from build123d import *

# Parameters (mm, degrees)
SKETCH2_R               = 3.175
BOSS_EXTRUDE2_DEPTH     = 3.81
SKETCH1_R               = 3.175
BOSS_EXTRUDE3_DEPTH     = 3.81
CUT_EXTRUDE1_DEPTH      = 130.839106153
CUT_EXTRUDE1_DEPTH_BACK = 130.839106153
SKETCH3_R               = 3.175


with BuildPart() as part:
    # Sketch2 → Boss-Extrude2 (new body)
    with BuildSketch(Plane(origin=(0, 0, 0), x_dir=(1, 0, 0), z_dir=(0, 1, 0))):
        with BuildLine():
            Line((-45.85683296, -6.1921984), (-122.640093118, 11.252530303))
            ThreePointArc((-122.640093118, 11.252530303), (-127.425458558, 18.851561662), (-119.826427198, 23.636927102))
            Line((-119.826427198, 23.636927102), (-43.04316704, 6.1921984))
            ThreePointArc((-43.04316704, 6.1921984), (-38.2578016, -1.40683296), (-45.85683296, -6.1921984))
        make_face()
        with Locations(Location((-121.233260158, 17.444728703, 0), (0, 0, 90))):
            Circle(SKETCH2_R, mode=Mode.SUBTRACT)
    extrude(amount=BOSS_EXTRUDE2_DEPTH)

    # Sketch1 → Boss-Extrude3 (add)
    with BuildSketch(Plane(origin=(0, 0, 0), x_dir=(1, 0, 0), z_dir=(0, 1, 0))):
        with BuildLine():
            Line((-44.45, 6.35), (44.45, 6.35))
            ThreePointArc((44.45, 6.35), (50.8, 0), (44.45, -6.35))
            Line((44.45, -6.35), (-44.45, -6.35))
            ThreePointArc((-44.45, -6.35), (-50.8, 0), (-44.45, 6.35))
        make_face()
        with Locations(Location((44.45, 0, 0), (0, 0, 90))):
            Circle(SKETCH1_R, mode=Mode.SUBTRACT)
    extrude(amount=BOSS_EXTRUDE3_DEPTH)

    # Sketch3 → Cut-Extrude1 (cut, two sides: drawn at the far end of the back side and taken through both)
    with BuildSketch(Plane(origin=(0, 3.81, 0), x_dir=(1, 0, 0), z_dir=(0, 1, 0)).offset(-CUT_EXTRUDE1_DEPTH_BACK)):
        with Locations(Location((-44.45, 0, 0), (0, 0, 270))):
            Circle(SKETCH3_R)
    extrude(amount=CUT_EXTRUDE1_DEPTH + CUT_EXTRUDE1_DEPTH_BACK, mode=Mode.SUBTRACT)


solid = part.part
Here's how the part is built. I have some questions about the finished solid (model axes, mm). A direction names the side the tool comes from. Coordinates: 2 decimals unless noted, no trailing zeros. Write each loop counter-clockwise with the first axis right and the second up, starting at its lowest first coordinate (ties: lowest second). Pieces come first, ordered by that corner, then holes.
Item 1: If I drill on line 1 (Z direction, x = 44.45, y = 1.35) (3 decimals); line 2 (Z direction, x = 39, y = 3.65); line 3 (Z direction, x = -72, y = 3.55), over which ranges is the centre line in solid material (lowest first)?
Item 2: On a 3-axis mill with a long thin cutter (end or side, diameter ignored), from which of +Z, -Z, +X, -X, +Y, -Y can I reach the whole of each face in a straight line? I mean faces 4 (the flat face through (0, 2, -6.35)), 5 (the flat face through (1, 2, 6.35)). Say none if no direction works.
Item 3: I want a section at A-A on z = 0. Write out the boundary of the cut face in (x, y) (3 decimals).
Item 4: Will these pins go through, and if not, where does the flat tip stop? pin 1 (1.1 mm diameter, centred on x = 9, y = 1, fed in from -Z); pin 2 (5 mm diameter, centred on x = 44.45, z = 0, fed in from +Y).
Item 5: I want a section at C-C on x = -16.5. Write out the boundary of the cut face in (y, z).
Item 6: If we mould it in two halves opening along X, with no side actions, what happens to faces 1 (the flat face through (-82.315, 1.878, -15.114)), 2 (the flat face through (-37, 3.81, -6)), 3 (the cylindrical face through (-41.3, 1.9, -0.4))? For each: +X half, -X half, draft (parallel to the pull), parting line (faces both ways), or undercut.
Item 7: I want a section at D-D on x = -75. Write out the boundary of the cut face in (y, z).
Item 8: I want a section at B-B on y = 2.8. Write out the boundary of the cut face in (x, z) (3 decimals), and give its area (3 significant figures).
Findings below:
1. line 1: z = -6.35 to -3.175, 3.175 to 6.35
1. line 2: z = -6.35 to 6.35
1. line 3: z = -12.77 to 0.25
2. face 4: -Z, +X, +Y, -Y
2. face 5: +Z, +X, -X, +Y, -Y
3. outline: (-73.112, 0) - (-47.625, 0) - (-47.625, 3.81) - (-73.112, 3.81) - close; (-41.275, 0) - (41.275, 0) - (41.275, 3.81) - (-41.275, 3.81) - close; (47.625, 0) - (50.8, 0) - (50.8, 3.81) - (47.625, 3.81) - close
4. pin 1: stops at z = -6.35
4. pin 2: passes through
5. outline: (0, -6.35) - (3.81, -6.35) - (3.81, 6.35) - (0, 6.35) - close
6. face 1: +X half
6. face 2: draft
6. face 3: undercut
7. outline: (0, -13.45) - (3.81, -13.45) - (3.81, -0.43) - (0, -0.43) - close
8. outline: (-122.64, -11.253) arc R6.35 ccw to (-119.826, -23.637) - (-43.738, -6.35) - (44.45, -6.35) arc R6.35 ccw to (44.45, 6.35) - (-44.45, 6.35) arc R6.35 ccw to (-45.857, 6.192) - close; hole circle Ø6.35 at (-121.233, -17.445); hole circle Ø6.35 at (-44.45, 0); hole circle Ø6.35 at (44.45, 0)
8. area: 2,160 mm2
